Part print with two shaded views. Sizes in mm from the minimum x, y, z corner. A direction names the side the tool comes from. Give positions to 0.01 mm unless a question says otherwise; leave off trailing zeros. Order: outer loops, then holes, each group sorted by start corner. A loop starts at its lowest first (then second) coordinate and runs counter-clockwise, first axis right, second up.
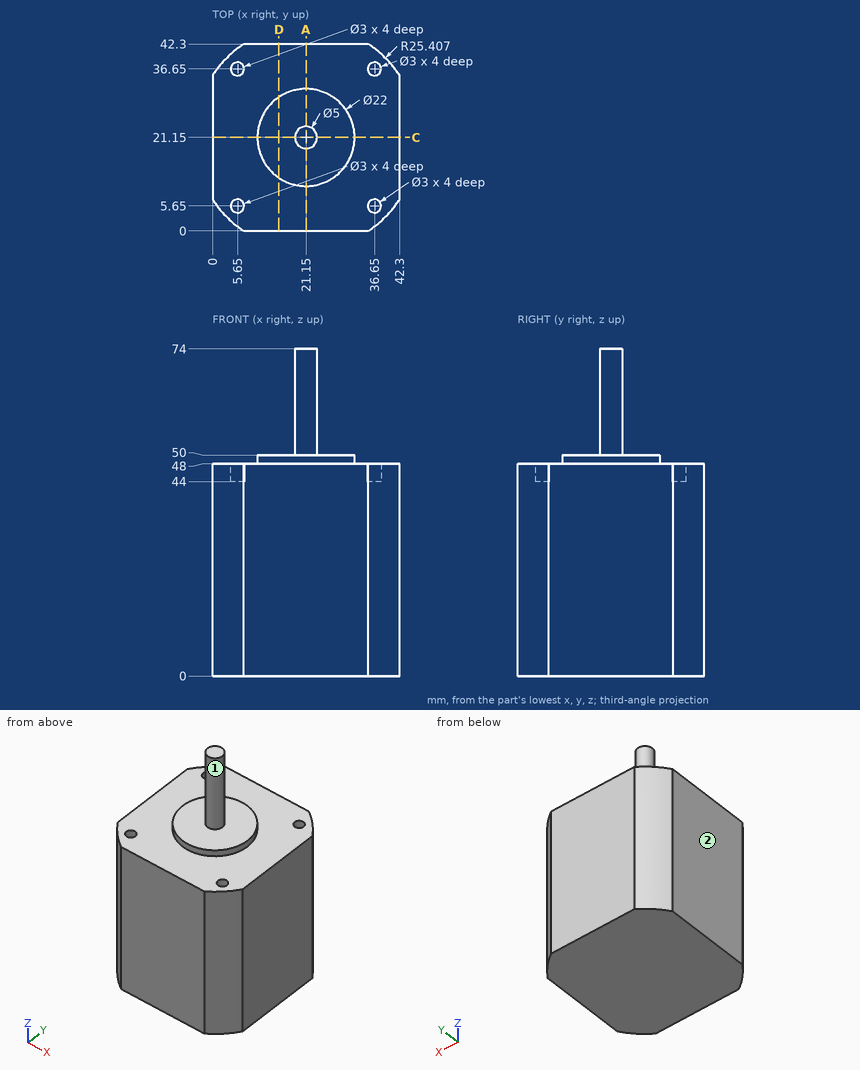
Item 1: Slice it at D-D (x = 15). Give the cut face in (y, z).
Item 2: Tool access for the marked faces 1 and 2: list every direction of +Z, -Z, +X, -X, +Y, -Y with a clear straight run to the whole face (end or side of a thin tool).
Item 3: Drop flat-ended pins along their axis: pin 1 Ø8 at (x, z) = (15.5, 30) entering from -Y; pin 2 Ø4 at (x, y) = (36.65, 5.65) entering from +Z; pin 3 Ø0.9 at (x, y) = (37, 6) entering from +Z; pin 4 Ø5 at (y, z) = (24.5, 53.5) entering from -X. Give the stop position or say it passes through.
Item 4: Slice it at A-A (x = 21.15). Give the cut face in (y, z), and give its area (3 significant figures).
Item 5: Wall check: L1, parallel to X at y = 5, z = 46 (1 decimal); L2, parallel to Z at x = 6.5, y = 22; L3, parallel to Z at x = 16.5, y = 14.5. Give the ranges that are in metal, low to high.
A:
1. outline: (0, 0) - (42.3, 0) - (42.3, 48) - (30.27, 48) - (30.27, 50) - (12.03, 50) - (12.03, 48) - (0, 48) - close
2. face 1: +Z
2. face 2: +Z, -Z, -X, +Y, -Y
3. pin 1: stops at y = 0
3. pin 2: stops at z = 48
3. pin 3: stops at z = 44
3. pin 4: stops at x = 18.8
4. outline: (0, 0) - (42.3, 0) - (42.3, 48) - (32.15, 48) - (32.15, 50) - (23.65, 50) - (23.65, 74) - (18.65, 74) - (18.65, 50) - (10.15, 50) - (10.15, 48) - (0, 48) - close
4. area: 2,190 mm2
5. L1: x = 1.5 to 4.3, 7 to 35.3, 38 to 40.8
5. L2: z = 0 to 48
5. L3: z = 0 to 50
